```python
from build123d import *

# Parameters (mm, degrees)
F0_W     = 35.56
F0_H     = 12.7
F1_DEPTH = 38.1
F2_DEPTH = 50.8
F4_DEPTH = 76.201
F5_DEPTH = 12.7
F6_DEPTH = 12.7


with BuildPart() as f1:
    # F0 (on Front) → F1 (new body)
    with BuildSketch(Plane.XZ):
        with Locations((38.1, 6.35)):
            Rectangle(F0_W, F0_H)
    extrude(amount=F1_DEPTH)

    # F0 (on Front) → F2 (join)
    with BuildSketch(Plane.XZ):
        Polygon((38.1, 38.1), (0, 0), (20.32, 0), (20.32, 12.7), (55.88, 12.7), (55.88, 0), (76.2, 0), align=None)
    extrude(amount=F2_DEPTH)

    # F3 (on Right) → F4 (cut, through all)
    with BuildSketch(Plane.YZ):
        Polygon((-50.8, 0), (0, 38.1), (-50.8, 38.1), align=None)
    extrude(amount=F4_DEPTH, mode=Mode.SUBTRACT)

    # F0 (on Front) → F5 (join)
    with BuildSketch(Plane.XZ):
        Polygon((0, 25.4), (0, 0), (38.1, 38.1), (76.2, 0), (76.2, 25.4), (50.8, 50.8), (25.4, 50.8), align=None)
    extrude(amount=-F5_DEPTH)

    # F0 (on Front) → F6 (join)
    with BuildSketch(Plane.XZ):
        with Locations((38.1, 6.35)):
            Rectangle(F0_W, F0_H)
        Polygon((0, 25.4), (0, 0), (38.1, 38.1), (76.2, 0), (76.2, 25.4), (50.8, 50.8), (25.4, 50.8), align=None)
        Polygon((38.1, 38.1), (0, 0), (20.32, 0), (20.32, 12.7), (55.88, 12.7), (55.88, 0), (76.2, 0), align=None)
    extrude(amount=-F6_DEPTH)


solid = f1.part
```
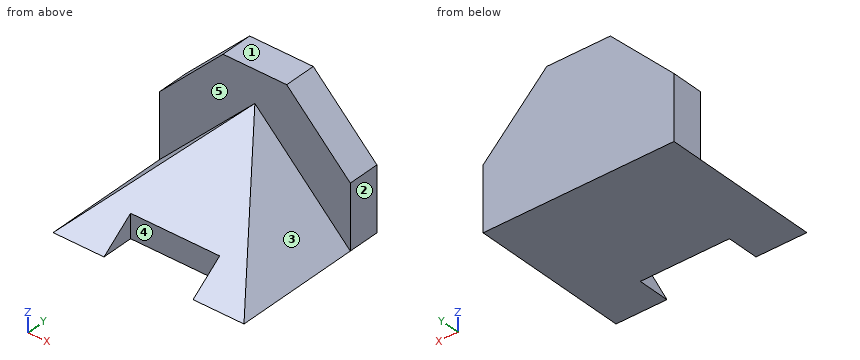
Here's how the part is built. I have some questions about the finished solid (model axes, mm). Face numbers are marked on the shaded views. A direction names the side the tool comes from. Coordinates: 2 decimals unless noted, no trailing zeros. Loops run counter-clockwise (first coordinate to the right, second up) from the corner with the lowest first, then second, coordinate; pieces in that order, holes last. Notation, with made-up numbers: (6.25, 44) - (10.25, 44) arc R22 cw to (10.25, 62) - close; hole circle Ø9 at (-32, 5.25). An arc over 180 degrees is marked (long way). Return JSON: item names as keys, results as strings. Group by question number.
Item 1: If we section it at C-C on z = 33: Write out the boundary of the cut face in (x, y).
Item 2: If we section it at B-B on y = -43.5: Write out the boundary of the cut face in (x, z) (3 decimals), and give its area (3 significant figures).
Item 3: I need wall thicknesses on line 1 (Y direction, x = 21.5, z = 9.5); line 2 (Y direction, x = 5.5, z = 22); line 3 (X direction, y = -20, z = 4). Which ranges of each line are inside material? Lowest first, please. Write a range as from..to.
Item 4: On a 3-axis mill with a long thin cutter (end or side, diameter ignored), from which of +Z, -Z, +X, -X, +Y, -Y can I reach the whole of each face in a straight line? I mean the marked faces 1, 2, 3, 4 and 5. Say none if no direction works.
Item 5: If we section it at A-A on x = 49.5: Write out the boundary of the cut face in (y, z) (3 decimals).
Item 6: Will these pins go through, and if not, where does the flat tip stop? P1, Ø15, axis at x = 56.5, z = 30.5, coming from the -Y side; P2, Ø3, axis at y = -47, z = 5, coming from the +X side; P3, Ø5, axis at x = 41.5, z = 4, coming from the -Y side; P4, Ø1.5, axis at x = 58.5, z = 6, coming from the -Y side.
Item 7: If we section it at D-D on y = -16: Write out the boundary of the cut face in (x, z), and give its area (3 significant figures).
Calculated:
{
 "1": {"outline": "(7.6, 0) - (33, 0) - (33, -6.8) - (43.2, -6.8) - (43.2, 0) - (68.6, 0) - (68.6, 12.7) - (7.6, 12.7) - close"},
 "2": {"outline": "(0, 0) - (20.32, 0) - (20.32, 5.475) - (5.475, 5.475) - close; (55.88, 0) - (76.2, 0) - (70.725, 5.475) - (55.88, 5.475) - close", "area": "193 mm^2"},
 "3": {"line 1": "y = -38.1..12.7", "line 2": "y = 0..12.7", "line 3": "x = 4..72.2"},
 "4": {"face 1": "+Z, +X, -X, +Y, -Y", "face 2": "+Z, -Z, +X, +Y, -Y", "face 3": "+Z, +X, -Y", "face 4": "+Z, -Z, -Y", "face 5": "+Z, -Y"},
 "5": {"outline": "(-38.1, 0) - (12.7, 0) - (12.7, 50.8) - (0, 50.8) - (0, 26.7) - (-15.2, 26.7) - (-38.1, 9.525) - close"},
 "6": {"P1": "stops at y = 0", "P2": "passes through", "P3": "stops at y = -38.1", "P4": "stops at y = -43.8"},
 "7": {"outline": "(0, 0) - (76.2, 0) - (50.1, 26.1) - (26.1, 26.1) - close", "area": "1,310 mm^2"}
}
